```python
from build123d import *

# Parameters (mm, degrees)
F0_W     = 10.16
F0_H     = 5.08
F0_W_2   = 3.2
F0_H_2   = 3.2
F1_DEPTH = 5.08
F2_W     = 4.572
F2_H     = 5.08
F3_DEPTH = 3.84
F4_R     = 1.5
F5_R     = 0.5


with BuildPart() as f1:
    # F0 (on Front) → F1 (new body)
    with BuildSketch(Plane.XZ):
        with Locations((14.68, 11.46)):
            Rectangle(F0_W, F0_H)
        with BuildLine():
            ThreePointArc((0, 1.27), (0.371974, 0.371974), (1.27, 0))
            Line((1.27, 0), (3.2, 0))
            Line((3.2, 0), (3.2, 3.2))
            Line((3.2, 3.2), (3.2, 10.8))
            Line((3.2, 10.8), (0, 10.8))
            Line((0, 10.8), (0, 1.27))
        make_face()
        with Locations((4.8, 1.6)):
            Rectangle(F0_W_2, F0_H_2)
        with BuildLine():
            Line((6.4, 3.2), (6.4, 0))
            Line((6.4, 0), (8.33, 0))
            ThreePointArc((8.33, 0), (9.228026, 0.371974), (9.6, 1.27))
            Line((9.6, 1.27), (9.6, 8.92))
            Line((9.6, 8.92), (9.6, 14))
            Line((9.6, 14), (6.4, 14))
            Line((6.4, 14), (6.4, 3.2))
        make_face()
        with BuildLine():
            Line((0, 0), (1.27, 0))
            ThreePointArc((1.27, 0), (0.371974, 0.371974), (0, 1.27))
            Line((0, 1.27), (0, 0))
        make_face()
        with BuildLine():
            ThreePointArc((9.6, 1.27), (9.228026, 0.371974), (8.33, 0))
            Line((8.33, 0), (9.6, 0))
            Line((9.6, 0), (9.6, 1.27))
        make_face()
        with BuildLine():
            Line((0, 12.73), (0, 10.8))
            Line((0, 10.8), (3.2, 10.8))
            Line((3.2, 10.8), (3.2, 14))
            Line((3.2, 14), (1.27, 14))
            ThreePointArc((1.27, 14), (0.371974, 13.628026), (0, 12.73))
        make_face()
        with BuildLine():
            Line((0, 14), (0, 12.73))
            ThreePointArc((0, 12.73), (0.371974, 13.628026), (1.27, 14))
            Line((1.27, 14), (0, 14))
        make_face()
    extrude(amount=F1_DEPTH)

    # F2 (on face) → F3 (join)
    with BuildSketch(Plane(origin=(0, 0, 8.92), x_dir=(1, 0, 0), z_dir=(0, 0, -1))):
        with Locations((17.474, 2.54)):
            Rectangle(F2_W, F2_H)
    extrude(amount=F3_DEPTH)

    # F4
    f4_edges = [f1.edges().sort_by_distance(p)[0] for p in [
        (0, -2.54, 0),
        (9.6, -2.54, 0),
        (0, -2.54, 14),
        (3.2, -2.54, 14),
        (6.4, -2.54, 14),
        (19.76, -2.54, 14),
        (19.76, -2.54, 5.08),
        (15.188, -2.54, 5.08),
    ]]
    fillet(f4_edges, radius=F4_R)

    # F5
    f5_edges = [f1.edges().sort_by_distance(p)[0] for p in [
        (6.4, -2.54, 3.2),
        (3.2, -2.54, 3.2),
        (15.188, -2.54, 8.92),
        (9.6, -2.54, 8.92),
    ]]
    fillet(f5_edges, radius=F5_R)


solid = f1.part
```
Work out the finished part from the listing and answer in its coordinate system (mm). A direction names the side the tool comes from. Round coordinates to 2 decimals unless told otherwise and drop trailing zeros. Write each loop counter-clockwise with the first axis right and the second up, starting at its lowest first coordinate (ties: lowest second). Pieces come first, ordered by that corner, then holes.
1) A cutting plane is placed at B-B on y = -3.35. Determine the outline of the cut face in (x, z), and give its area (3 significant figures).
2) Consider probe 1 along X at (y, z) = (-3.5, 6.5); probe 2 along X at (y, z) = (-4.4, 10); probe 3 along X at (y, z) = (-0.4, 4.5). Determine where each line is inside the solid, lowest interval first.
3) Which of the six approach directions +Z, -Z, +X, -X, +Y, -Y give full straight-line access (tool end or side, diameter ignored) to faces 4 (the face through (6.4, -3, 8)), 5 (the face through (9.15, -2.58, 0.43)), 6 (the face through (15.616, -2.576, 5.531))?
4) A cutting plane is placed at A-A on z = 4.25. Determine the outline of the cut face in (x, y).
5) A cutting plane is placed at D-D on x = 12.5. Determine the outline of the cut face in (y, z), and give its area (3 significant figures).
6) A cutting plane is placed at C-C on z = 12.25. Determine the outline of the cut face in (x, y).
7) Determine the mould class of faces 1 (the face through (6.85, -2.58, 13.57)), 2 (the face through (19.76, -3, 10)), 3 (the face through (17, -3, 5.08)) for opening direction X: pulls with the +X half, pulls with the -X half, needs draft (parallel to the pull), parting line crosses it, or undercut.
8) Flat-ended cylindrical pins translate along their axes: P1, Ø2.5, axis at x = 12, y = -2.5, coming from the -Z side; P2, Ø0.8, axis at x = 17.5, y = -3.5, coming from the -Z side; P3, Ø2.5, axis at x = 5, y = -3, coming from the +Z side; P4, Ø8, axis at x = 4, z = 6.5, coming from the +Y side. Find the tip coordinate at first contact, or state that the pin passes through.
Entries:
1. outline: (0, 1.5) arc R1.5 ccw to (1.5, 0) - (8.1, 0) arc R1.5 ccw to (9.6, 1.5) - (9.6, 8.42) arc R0.5 cw to (10.1, 8.92) - (14.69, 8.92) arc R0.5 cw to (15.19, 8.42) - (15.19, 6.58) arc R1.5 ccw to (16.69, 5.08) - (18.26, 5.08) arc R1.5 ccw to (19.76, 6.58) - (19.76, 12.5) arc R1.5 ccw to (18.26, 14) - (7.9, 14) arc R1.5 ccw to (6.4, 12.5) - (6.4, 3.7) arc R0.5 cw to (5.9, 3.2) - (3.7, 3.2) arc R0.5 cw to (3.2, 3.7) - (3.2, 12.5) arc R1.5 ccw to (1.7, 14) - (1.5, 14) arc R1.5 ccw to (0, 12.5) - close
1. area: 165 mm2
2. probe 1: x = 0 to 3.2, 6.4 to 9.6, 15.19 to 19.76
2. probe 2: x = 0 to 3.2, 6.4 to 19.76
2. probe 3: x = 0 to 3.2, 6.4 to 9.6
3. face 4: +Z, +Y, -Y
3. face 5: -Z, +X, +Y, -Y
3. face 6: -Z, +Y, -Y
4. outline: (0, -5.08) - (3.2, -5.08) - (3.2, 0) - (0, 0) - close; (6.4, -5.08) - (9.6, -5.08) - (9.6, 0) - (6.4, 0) - close
5. outline: (-5.08, 8.92) - (0, 8.92) - (0, 14) - (-5.08, 14) - close
5. area: 25.8 mm2
6. outline: (0, -5.08) - (3.2, -5.08) - (3.2, 0) - (0, 0) - close; (6.4, -5.08) - (19.76, -5.08) - (19.76, 0) - (6.4, 0) - close
7. face 1: undercut
7. face 2: pulls with the +X half
7. face 3: needs draft
8. P1: stops at z = 8.92
8. P2: stops at z = 5.08
8. P3: stops at z = 3.34
8. P4: stops at y = 0
